```python
from build123d import *
from build123d.topology import SkipClean

# Parameters (mm, degrees)
SKETCH1_R           = 15
BOSS_EXTRUDE1_DEPTH = 48
BOSS_EXTRUDE3_DEPTH = 6.9
BOSS_EXTRUDE4_START = 10
BOSS_EXTRUDE4_DEPTH = 10
SKETCH2_5_W         = 20
SKETCH2_5_H         = 6
CUT_EXTRUDE1_DEPTH  = 82.633326528
SKETCH3_R           = 4
CUT_EXTRUDE2_DEPTH  = 10


with BuildPart() as part:
    # Sketch1 → Boss-Extrude1 (new body)
    with BuildSketch(Plane.XY):
        with BuildLine():
            Line((-22, 0), (-22, -37.999983616))
            Line((-22, -37.999983616), (-16.5, -37.999983616))
            Line((-16.5, -37.999983616), (-16.5, -23))
            Line((-16.5, -23), (16.5, -23))
            Line((16.5, -23), (16.5, -38))
            Line((16.5, -38), (22, -38))
            Line((22, -38), (22, 0))
            ThreePointArc((22, 0), (0, 22), (-22, 0))
        make_face()
        Circle(SKETCH1_R, mode=Mode.SUBTRACT)
    boss_extrude1 = extrude(amount=-BOSS_EXTRUDE1_DEPTH)

    # Sketch2 → Boss-Extrude3 (add)
    with BuildSketch(Plane(origin=(22, 0, 0), x_dir=(0, 0, -1), z_dir=(1, 0, 0))):
        with BuildLine():
            Line((7, 16), (7, 0))
            Line((7, 0), (14, 0))
            ThreePointArc((14, 0), (16.928932188, 7.071067812), (24, 10))
            Line((24, 10), (24, 16))
            Line((24, 16), (7, 16))
        make_face()
        with BuildLine():
            Line((41, 16), (24, 16))
            Line((24, 16), (24, 10))
            ThreePointArc((24, 10), (31.071067812, 7.071067812), (34, 0))
            Line((34, 0), (41, 0))
            Line((41, 0), (41, 16))
        make_face()
    boss_extrude3 = extrude(amount=-BOSS_EXTRUDE3_DEPTH)

    # Sketch2<4> → Boss-Extrude4 (add)
    with BuildSketch(Plane(origin=(22, 0, 0), x_dir=(0, 0, -1), z_dir=(1, 0, 0)).offset(BOSS_EXTRUDE4_START)):
        with BuildLine():
            Line((41, 16), (24, 16))
            Line((24, 16), (24, 10))
            ThreePointArc((24, 10), (31.071067812, 7.071067812), (34, 0))
            Line((34, 0), (41, 0))
            Line((41, 0), (41, 16))
        make_face()
        with BuildLine():
            Line((7, 16), (7, 0))
            Line((7, 0), (14, 0))
            ThreePointArc((14, 0), (16.928932188, 7.071067812), (24, 10))
            Line((24, 10), (24, 16))
            Line((24, 16), (7, 16))
        make_face()
        with BuildLine():
            Line((7, 0), (7, -38))
            Line((7, -38), (14, -38))
            Line((14, -38), (14, -32))
            Line((14, -32), (24, -32))
            Line((24, -32), (24, -10))
            ThreePointArc((24, -10), (16.928932188, -7.071067812), (14, 0))
            Line((14, 0), (7, 0))
        make_face()
        with BuildLine():
            Line((34, -32), (34, -38))
            Line((34, -38), (41, -38))
            Line((41, -38), (41, 0))
            Line((41, 0), (34, 0))
            ThreePointArc((34, 0), (31.071067812, -7.071067812), (24, -10))
            Line((24, -10), (24, -32))
            Line((24, -32), (34, -32))
        make_face()
    boss_extrude4 = extrude(amount=-BOSS_EXTRUDE4_DEPTH)

    # Mirror2: Boss-Extrude1, Boss-Extrude3, Boss-Extrude4 across plane
    add(boss_extrude1.mirror(Plane.ZY))
    add(boss_extrude3.mirror(Plane.ZY))
    add(boss_extrude4.mirror(Plane.ZY))

    # Sketch2<5> → Cut-Extrude1 (cut, through all)
    with SkipClean():  # the faces are left unmerged after this step: merging them gives an invalid solid
        with BuildSketch(Plane(origin=(22, 0, 0), x_dir=(0, 0, -1), z_dir=(1, 0, 0))):
            with BuildLine():
                Line((24, 0), (14, 0))
                ThreePointArc((14, 0), (16.928932188, -7.071067812), (24, -10))
                Line((24, -10), (24, 0))
            make_face()
            with BuildLine():
                ThreePointArc((24, 10), (16.928932188, 7.071067812), (14, 0))
                Line((14, 0), (24, 0))
                Line((24, 0), (24, 10))
            make_face()
            with BuildLine():
                ThreePointArc((34, 0), (31.071067812, 7.071067812), (24, 10))
                Line((24, 10), (24, 0))
                Line((24, 0), (34, 0))
            make_face()
            with BuildLine():
                Line((24, 0), (24, -10))
                ThreePointArc((24, -10), (31.071067812, -7.071067812), (34, 0))
                Line((34, 0), (24, 0))
            make_face()
            with Locations((24, -35)):
                Rectangle(SKETCH2_5_W, SKETCH2_5_H)
        extrude(amount=-CUT_EXTRUDE1_DEPTH, mode=Mode.SUBTRACT)

    # Sketch3 → Cut-Extrude2 (cut)
    with SkipClean():  # the faces are left unmerged after this step: merging them gives an invalid solid
        with BuildSketch(Plane(origin=(0, 16, 0), x_dir=(1, 0, 0), z_dir=(0, 1, 0))):
            with Locations(Location((24, 24, 0), (0, 0, 180))):
                Circle(SKETCH3_R)
            with Locations(Location((-24, 24, 0), (0, 0, 180))):
                Circle(SKETCH3_R)
        extrude(amount=-CUT_EXTRUDE2_DEPTH, mode=Mode.SUBTRACT)


solid = part.part
```
The model under review builds one solid part; all positions refer to its coordinate system, in mm. A direction names the side the tool comes from. Give positions to 0.01 mm unless a question says otherwise; leave off trailing zeros. Write each loop counter-clockwise with the first axis right and the second up, starting at its lowest first coordinate (ties: lowest second). Pieces come first, ordered by that corner, then holes. Notation, with made-up numbers: (-7, 12) - (26, 12) arc R30 ccw to (26, 34) - close; hole circle Ø10 at (-26.5, -4). An arc over 180 degrees is marked (long way). Answer in a Markdown table with one row per item. Add a question column.
1. Insertion check: P1, Ø5.5, axis at y = -12, z = -2.5, coming from the -X side; P2, Ø1.8, axis at x = -27.5, y = -34, coming from the -Z side; P3, Ø13.5, axis at x = 25.5, z = -17.5, coming from the +Y side; P4, Ø12, axis at y = 0, z = -24, coming from the +X side. Each pin has a flat end and moves straight along its axis. Give the tip position at first contact, or say it passes through.
2. Draft analysis for pull direction X (two halves, no side actions). For faces 6 (the flat face through (22, 16, -28)), 7 (the flat face through (16.5, -30, -24)), 8 (the flat face through (22, -19, -3)), state which applies: +X half, -X half, draft (parallel to the pull), parting line (faces both ways), or undercut.
3. Wall thickness on line 1 along Z through (x, y) = (-24, 12.5); line 2 along X through (y, z) = (-10, -36); line 3 along Z through (x, y) = (24.75, 0): over which ranges is each line inside the solid? List them lowest first. Write a range as [from, to].
4. We need section B-B on x = 0. Write out the cut boundary in (y, z).
5. We need section D-D on x = -24. Write out the cut boundary in (y, z), then the cut area to 3 significant figures.
6. We need section A-A on y = -24.5. Write out the cut boundary in (x, z), then the cut area to 3 significant figures.
7. Tool access review of faces 1 (the flat face through (-22, 16, -28)), 2 (the cylindrical face through (20.305, 12.63, -25.532)), 3 (the flat face through (22, -19, -44)), 4 (the flat face through (0, -23, -24)), 5 (the flat face through (-22, -19, -44)): name each direction out of +Z, -Z, +X, -X, +Y, -Y from which nothing blocks a thin tool from reaching the whole face with its end or side.
Ans:
| question | item | result |
|---|---|---|
| 1 | P1 | stops at x = -22 |
| 1 | P2 | stops at z = -41 |
| 1 | P3 | stops at y = 16 |
| 1 | P4 | passes through |
| 2 | face 6 | draft |
| 2 | face 7 | undercut |
| 2 | face 8 | +X half |
| 3 | line 1 | z = [-41, -28], [-20, -7] |
| 3 | line 2 | x = [-32, -11.18], [11.18, 32] |
| 3 | line 3 | z = [-41, -34], [-14, -7] |
| 4 | outline | (-23, -48) - (-15, -48) - (-15, 0) - (-23, 0) - close; (15, -48) - (22, -48) - (22, 0) - (15, 0) - close |
| 5 | outline | (-38, -41) - (16, -41) - (16, -28) - (9.17, -28) arc R10 cw (long way) to (9.17, -20) - (16, -20) - (16, -7) - (-38, -7) - (-38, -14) - (-32, -14) - (-32, -34) - (-38, -34) - close |
| 5 | area | 1,350 mm^2 |
| 6 | outline | (-32, -41) - (-22, -41) - (-22, -48) - (-16.5, -48) - (-16.5, 0) - (-22, 0) - (-22, -7) - (-32, -7) - close; (16.5, -48) - (22, -48) - (22, -41) - (32, -41) - (32, -7) - (22, -7) - (22, 0) - (16.5, 0) - close |
| 6 | area | 1,210 mm^2 |
| 7 | face 1 | +Z, -Z, -X, +Y |
| 7 | face 2 | +Y |
| 7 | face 3 | -Z, +X, +Y, -Y |
| 7 | face 4 | +Z, -Z, -Y |
| 7 | face 5 | -Z, -X, +Y, -Y |
